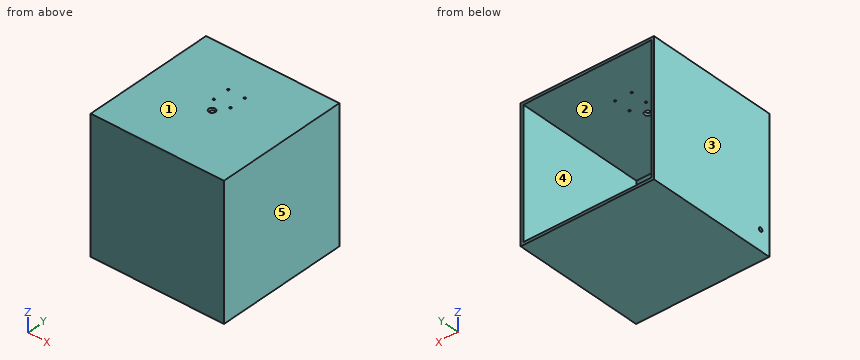
```python
from build123d import *

# Parameters (mm, degrees)
SKETCH1_W           = 200
SKETCH1_H           = 200
BOSS_EXTRUDE1_DEPTH = 200
SHELL1_T            = -4
CUT_EXTRUDE1_REACH  = 302
SKETCH2_R           = 1.5
SKETCH2_R_2         = 5
CUT_EXTRUDE2_REACH  = 302
SKETCH3_R           = 3


with BuildPart() as part:
    # Sketch1 → Boss-Extrude1 (new body)
    with BuildSketch(Plane(origin=(0, 0, 0), x_dir=(1, 0, 0), z_dir=(0, 1, 0))):
        Rectangle(SKETCH1_W, SKETCH1_H)
    extrude(amount=BOSS_EXTRUDE1_DEPTH)

    # Shell1
    shell1_openings = [part.faces().sort_by_distance(p)[0] for p in [
        (0, 200, 0),
    ]]
    offset(amount=SHELL1_T, openings=shell1_openings, kind=Kind.INTERSECTION)

    # Sketch2 → Cut-Extrude1 (cut, up to next)
    with BuildSketch(Plane.XY.offset(100), mode=Mode.PRIVATE) as cut_extrude1_sk1:
        with Locations((-12.5, 137.5)):
            Circle(SKETCH2_R)
    cut_extrude1_tool1 = extrude(cut_extrude1_sk1.sketch, amount=-CUT_EXTRUDE1_REACH, mode=Mode.PRIVATE) & part.part
    # Sketch2 → Cut-Extrude1 (cut, up to next)
    with BuildSketch(Plane.XY.offset(100), mode=Mode.PRIVATE) as cut_extrude1_sk2:
        with Locations((12.5, 137.5)):
            Circle(SKETCH2_R)
    cut_extrude1_tool2 = extrude(cut_extrude1_sk2.sketch, amount=-CUT_EXTRUDE1_REACH, mode=Mode.PRIVATE) & part.part
    # Sketch2 → Cut-Extrude1 (cut, up to next)
    with BuildSketch(Plane.XY.offset(100), mode=Mode.PRIVATE) as cut_extrude1_sk3:
        with Locations((12.5, 112.5)):
            Circle(SKETCH2_R)
    cut_extrude1_tool3 = extrude(cut_extrude1_sk3.sketch, amount=-CUT_EXTRUDE1_REACH, mode=Mode.PRIVATE) & part.part
    # Sketch2 → Cut-Extrude1 (cut, up to next)
    with BuildSketch(Plane.XY.offset(100), mode=Mode.PRIVATE) as cut_extrude1_sk4:
        with Locations((-12.5, 112.5)):
            Circle(SKETCH2_R)
    cut_extrude1_tool4 = extrude(cut_extrude1_sk4.sketch, amount=-CUT_EXTRUDE1_REACH, mode=Mode.PRIVATE) & part.part
    # Sketch2 → Cut-Extrude1 (cut, up to next)
    with BuildSketch(Plane.XY.offset(100), mode=Mode.PRIVATE) as cut_extrude1_sk5:
        with Locations((0, 95)):
            Circle(SKETCH2_R_2)
    cut_extrude1_tool5 = extrude(cut_extrude1_sk5.sketch, amount=-CUT_EXTRUDE1_REACH, mode=Mode.PRIVATE) & part.part
    add(cut_extrude1_tool1.solids().sort_by_distance((-12.5, 137.5, 100))[0], mode=Mode.SUBTRACT)
    add(cut_extrude1_tool2.solids().sort_by_distance((12.5, 137.5, 100))[0], mode=Mode.SUBTRACT)
    add(cut_extrude1_tool3.solids().sort_by_distance((12.5, 112.5, 100))[0], mode=Mode.SUBTRACT)
    add(cut_extrude1_tool4.solids().sort_by_distance((-12.5, 112.5, 100))[0], mode=Mode.SUBTRACT)
    add(cut_extrude1_tool5.solids().sort_by_distance((0, 95, 100))[0], mode=Mode.SUBTRACT)

    # Sketch3 → Cut-Extrude2 (cut, up to next)
    with BuildSketch(Plane.ZY.offset(100), mode=Mode.PRIVATE) as cut_extrude2_sk1:
        with Locations((-70, 15)):
            Circle(SKETCH3_R)
    cut_extrude2_tool1 = extrude(cut_extrude2_sk1.sketch, amount=-CUT_EXTRUDE2_REACH, mode=Mode.PRIVATE) & part.part
    add(cut_extrude2_tool1.solids().sort_by_distance((-100, 15, -70))[0], mode=Mode.SUBTRACT)


solid = part.part
```
Can you work these out from the model? Positions are in its coordinate system, mm. Face numbers are marked on the shaded views. A direction names the side the tool comes from. Coordinates: 2 decimals unless noted, no trailing zeros. Write each loop counter-clockwise with the first axis right and the second up, starting at its lowest first coordinate (ties: lowest second). Pieces come first, ordered by that corner, then holes. Notation, with made-up numbers: M 22.5,-29 L 28.5,-29 A5 cw 28.5,-20 Z; hole C 76.5,-37.75 d1. An arc over 180 degrees is marked long. Answer as CSV lines item,"result".
Item 1: On a 3-axis mill with a long thin cutter (end or side, diameter ignored), from which of +Z, -Z, +X, -X, +Y, -Y can I reach the whole of each face in a straight line? I mean the marked faces 4 and 5. Say none if no direction works.
Geometry results:
face 4,"+Y"
face 5,"+Z, -Z, +X, +Y, -Y"
Item 2: Imagine slicing it at C-C on y = 77. List the corners of the cut face in (x, z) for me, plus the area to 3 significant figures.
Geometry results:
outline,"M -100,-100 L 100,-100 L 100,100 L -100,100 Z; hole M -96,-96 L 96,-96 L 96,96 L -96,96 Z"
area,"3,140 mm2"
Item 3: Please list where these lines run through material, in increasing order: line 1 along X through (y, z) = (137.5, 98.2); line 2 along Y through (x, z) = (-12.5, 97.8); line 3 along Z through (x, y) = (-78, 39.5).
Geometry results:
line 1,"x = -100 to -14, -11 to 11, 14 to 100"
line 2,"y = 0 to 111, 114 to 136, 139 to 200"
line 3,"z = -100 to -96, 96 to 100"
Item 4: We'd pull the mould along Z, two halves only. Please class the marked faces 1, 2 and 3: +Z half, -Z half, draft (parallel to the pull), parting line (faces both ways), or undercut.
Geometry results:
face 1,"+Z half"
face 2,"undercut"
face 3,"draft"
Item 5: Imagine slicing it at A-A on x = 0. List the corners of the cut face in (y, z) for me.
Geometry results:
outline,"M 0,-100 L 200,-100 L 200,-96 L 4,-96 L 4,96 L 90,96 L 90,100 L 0,100 Z; M 100,96 L 200,96 L 200,100 L 100,100 Z"
Item 6: Imagine slicing it at D-D on x = -79. List the corners of the cut face in (y, z) for me.
Geometry results:
outline,"M 0,-100 L 200,-100 L 200,-96 L 4,-96 L 4,96 L 200,96 L 200,100 L 0,100 Z"
Item 7: I'm going to push flat-ended pins straight in: P1, Ø4, axis at x = 27.5, z = -34, coming from the +Y side; P2, Ø2.5, axis at x = 12.5, y = 137.5, coming from the +Z side. Where does each tip first touch, or does it pass through?
Geometry results:
P1,"stops at y = 4"
P2,"stops at z = -96"
Item 8: Imagine slicing it at B-B on z = -41.5. List the corners of the cut face in (x, y) for me, plus the area to 3 significant figures.
Geometry results:
outline,"M -100,0 L 100,0 L 100,200 L 96,200 L 96,4 L -96,4 L -96,200 L -100,200 Z"
area,"2,370 mm2"
